Autodesk Inventor part; units mm, degrees
ref_plane "YZ Plane" through (0, 0, 0) normal (1, 0, 0) x (0, 1, 0)
ref_plane "XZ Plane" through (0, 0, 0) normal (0, 1, 0) x (-1, 0, 0)
ref_plane "XY Plane" through (0, 0, 0) normal (0, 0, 1) x (1, 0, 0)
sketch "草圖1" plane through (0, 0, 0) normal (0, 1, 0) x (-1, 0, 0)
  circle A0 centre (0, 0) radius 20
  line L0 (0, -20) -> (-30, -20)
  line L1 (-30, -20) -> (-30, 20)
  line L2 (-30, 20) -> (0, 20)
  line L3 (0, 20) -> (0, -20)
  point P0 (0, 20)
  dimension "d0" = 40
  dimension "d1" = 30
extrude "擠出1" add sketch "草圖1" along normal blind 40
sketch "草圖2" plane through (0, 40, 0) normal (0, 1, 0) x (1, 0, 0)
  line L0 (30, -20) -> (0, -20)
  arc A0 (0, 20) -> (0, -20) centre (0, 0) ccw
  line L1 (0, 20) -> (30, 20)
  line L2 (30, 20) -> (30, -20)
  line L3 (10, 20) -> (30, 20)
  line L4 (30, 20) -> (30, -20)
  line L5 (30, -20) -> (10, -20)
  line L6 (10, -20) -> (10, 20)
  line L7 (30, -20) -> (30, 20)
  line L8 (30, 20) -> (0, 20)
  line L9 (0, -20) -> (30, -20)
  line L10 (0, 10) -> (10, 10)
  line L11 (10, 10) -> (10, -10)
  line L12 (10, -10) -> (0, -10)
  line L13 (0, -10) -> (0, 10)
  circle A1 centre (0, 0) radius 10
  point P0 (10, 0)
  point P1 (0, -10)
  dimension "d4" = 20
  dimension "d5" = 20
  dimension "d6" = 10
extrude "擠出2" cut sketch "草圖2" against normal blind 20 contours L0 L6 L1 L2 | L12 A1 L6 | A1 L10 L6 | A1 L13 | A1 L13
sketch "草圖3" plane through (0, 20, 0) normal (0, 1, 0) x (1, 0, 0)
  line L0 (10, 20) -> (10, 10)
  line L1 (10, 10) -> (0, 10)
  arc A0 (0, 10) -> (0, -10) centre (0, 0) ccw
  line L2 (0, -10) -> (10, -10)
  line L3 (10, -10) -> (10, -20)
  line L4 (30, -20) -> (10, -20)
  line L5 (30, 20) -> (30, -20)
  line L6 (10, 20) -> (30, 20)
  line L7 (0, 20) -> (10, 20)
  arc A1 (0, 20) -> (0, -20) centre (0, 0) ccw
  line L8 (10, -20) -> (0, -20)
  circle A2 centre (30, 0) radius 10
  dimension "d9" = 20
extrude "擠出3" cut sketch "草圖3" against normal through all contours A2 L5 | L5 A2
properties part number "29" material "鋼、碳鋼"
Input: part model. Units: mm. Frame: model coordinates. A direction names the side the tool comes from. Coordinates: 2 decimals unless noted, no trailing zeros. Write each loop counter-clockwise with the first axis right and the second up, starting at its lowest first coordinate (ties: lowest second). Pieces come first, ordered by that corner, then holes. Notation, with made-up numbers: (-11, 27) -> (12, 27) arc R23 ccw to (12, 52) -> close; hole circle Ø11 at (57.25, -20.5). An arc over 180 degrees is marked (long way). Answer as a JSON object with one key per item and string values.
1. First-contact query: P1, Ø3, axis at x = 20.5, z = 1, coming from the -Y side; P2, Ø10, axis at y = 22, z = -9.5, coming from the -X side; P3, Ø3, axis at x = -6, y = 18, coming from the -Z side; P4, Ø1.5, axis at x = -13, y = 4.5, coming from the +Z side. Flat tips, straight axial feed; report the tip coordinate or a pass-through.
Result set:
{"P1": "stops at y = 0", "P2": "stops at x = -19.49", "P3": "stops at z = -19.49", "P4": "stops at z = 15.81"}
2. Section C-C on z = 0. Return the cut outline in (x, y), then the cut area to 3 significant figures.
Result set:
{"outline": "(-20, 0) -> (20, 0) -> (20, 20) -> (-10, 20) -> (-10, 40) -> (-20, 40) -> close", "area": "1,000 mm2"}
3. Section D-D on y = 10.5. Return the cut outline in (x, z).
Result set:
{"outline": "(0, -20) -> (30, -20) -> (30, -10) arc R10 cw to (30, 10) -> (30, 20) -> (0, 20) arc R20 ccw to start"}
4. Mould query, pull axis Z, two halves, no side actions, for faces 4 (the face through (-20, 20, 0)), 5 (the face through (10, 20, 0)), 6 (the face through (30, 10, 15)). Classes: released by +Z, released by -Z, zero draft, split by the parting line, or undercut.
Result set:
{"face 4": "split by the parting line", "face 5": "undercut", "face 6": "zero draft"}
5. Material intervals for line 1 (Z direction, x = 6, y = 35); line 2 (Y direction, x = 12.5, z = 10); line 3 (Z direction, x = -2.5, y = 26), sorted ascending. Write a range as from..to.
Result set:
{"line 1": "z = -20..-10, 10..20", "line 2": "y = 0..20", "line 3": "z = -19.84..-9.68, 9.68..19.84"}
6. Access query for faces 1 (the face through (10, 30, -15)), 2 (the face through (5, 0, 0)), 3 (the face through (5, 30, 10)). Directions: +Z, -Z, +X, -X, +Y, -Y. A direction counts if a zero-diameter tool reaches every point of the face in a straight line with its end or side. Return the directions, or none.
Result set:
{"face 1": "+Z, -Z, +X, +Y", "face 2": "+Z, -Z, +X, -X, -Y", "face 3": "+X, +Y"}
7. Section A-A on y = 29. Return the cut outline in (x, z), then the cut area to 3 significant figures.
Result set:
{"outline": "(0, -20) -> (10, -20) -> (10, -10) -> (0, -10) arc R10 cw to (0, 10) -> (10, 10) -> (10, 20) -> (0, 20) arc R20 ccw to start", "area": "671 mm2"}
8. Section B-B on x = 1.5. Return the cut outline in (y, z).
Result set:
{"outline": "(0, -20) -> (40, -20) -> (40, -10) -> (20, -10) -> (20, 10) -> (40, 10) -> (40, 20) -> (0, 20) -> close"}
